Answer from the drawing. Dimensions are ordinates in mm from the lowest x, y and z of the part. Round coordinates to 2 decimals unless told otherwise and drop trailing zeros. Write each loop counter-clockwise with the first axis right and the second up, starting at its lowest first coordinate (ties: lowest second). Pieces come first, ordered by that corner, then holes. Notation, with made-up numbers: (23, 87) - (72, 87) arc R12 cw to (72, 95) - close; hole circle Ø3 at (20, 33.5). An arc over 180 degrees is marked (long way). Write item = value, one per line. Start each with the question number.
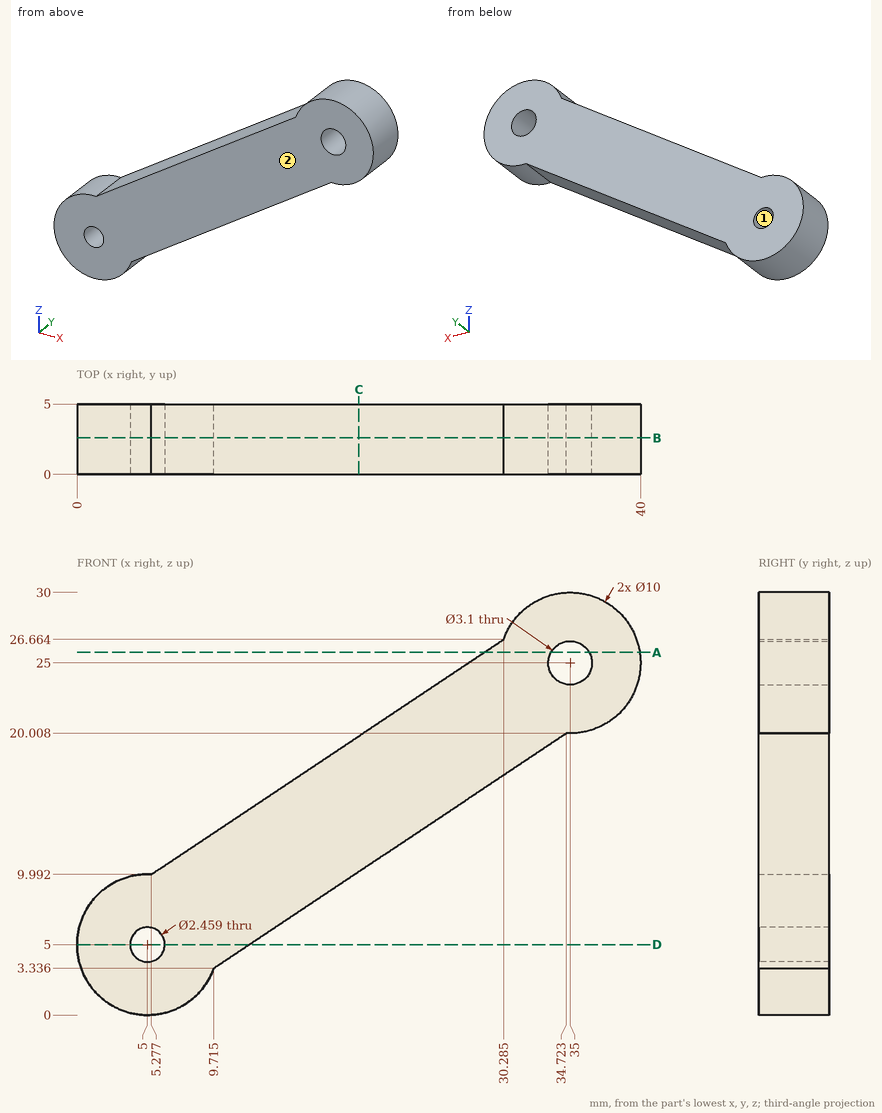
1. Find section A-A on z = 25.75. Give the vertices of the cut face in (x, y).
2. Find section D-D on z = 5. Give the vertices of the cut face in (x, y).
3. Consider line 1 (Z direction, x = 35, y = 3.4); line 2 (Z direction, x = 5, y = 1.9); line 3 (X direction, y = 3.3, z = 25). Determine where each line is inside the solid, lowest interval first.
4. Find section C-C on x = 20. Give the vertices of the cut face in (y, z), plus the area to 3 significant figures.
5. For a pull along X with two mould halves and no side action, classify the marked faces 1 and 2 as released by +X, released by -X, zero draft, split by the parting line, or undercut.
6. Each of these flat-tipped pins is pushed along its axis until it touches: pin 1 (3 mm diameter, centred on x = 10.5, y = 0.5, fed in from +Z) (1 decimal); pin 2 (2 mm diameter, centred on x = 9, y = 1, fed in from -Z); pin 3 (1 mm diameter, centred on y = 0.5, z = 7, fed in from +X). Where does it stop, or does it pass through?
7. Find section B-B on y = 2.6. Give the number of separate pieces and of enclosed holes in the cut face, plus the area to 3 significant figures.
Answer key:
q1.outline = (28.91, 0) - (33.64, 0) - (33.64, 5) - (28.91, 5) - close; (36.36, 0) - (39.94, 0) - (39.94, 5) - (36.36, 5) - close
q2.outline = (0, 0) - (3.77, 0) - (3.77, 5) - (0, 5) - close; (6.23, 0) - (12.21, 0) - (12.21, 5) - (6.23, 5) - close
q3.line_1 = 20 to 23.45, 26.55 to 30
q3.line_2 = 0 to 3.77, 6.23 to 10
q3.line_3 = 27.79 to 33.45, 36.55 to 40
q4.outline = (0, 10.19) - (5, 10.19) - (5, 19.81) - (0, 19.81) - close
q4.area = 48.1 mm²
q5.face_1 = undercut
q5.face_2 = zero draft
q6.pin_1 = 14.5
q6.pin_2 = 1
q6.pin_3 = 15.96
q7.separate_pieces = 1
q7.enclosed_holes = 2
q7.area = 363 mm²
